For this review, take the finished solid that the model builds, in its own axes (mm). A direction names the side the tool comes from. Round coordinates to 2 decimals unless told otherwise and drop trailing zeros. Write each loop counter-clockwise with the first axis right and the second up, starting at its lowest first coordinate (ties: lowest second). Pieces come first, ordered by that corner, then holes. Notation, with made-up numbers: M 60.5,85.5 L 75.5,85.5 A20 cw 75.5,115.5 Z; hole C -4,87 d5. An arc over 180 degrees is marked long. Answer in a Markdown table with one row per item.
```python
from build123d import *

# Parameters (mm, degrees)
SKETCH1_R           = 20.32
BOSS_EXTRUDE1_DEPTH = 26.416
BOSS_EXTRUDE2_DEPTH = 6.35
SKETCH3_R           = 12.7
BOSS_EXTRUDE3_DEPTH = 19.05
SKETCH4_R           = 2.032
CUT_EXTRUDE1_DEPTH  = 10.16


with BuildPart() as part:
    # Sketch1 → Boss-Extrude1 (new body)
    with BuildSketch(Plane(origin=(0, 0, 0), x_dir=(1, 0, 0), z_dir=(0, 1, 0))):
        Circle(SKETCH1_R)
    extrude(amount=BOSS_EXTRUDE1_DEPTH)

    # Sketch2 → Boss-Extrude2 (add)
    with BuildSketch(Plane.XZ):
        Polygon((-11.878404438, 20.574), (11.878404438, 20.574), (23.756808877, 0), (11.878404438, -20.574), (-11.878404438, -20.574), (-23.756808877, 0), align=None)
    extrude(amount=BOSS_EXTRUDE2_DEPTH)

    # Sketch3 → Boss-Extrude3 (add)
    with BuildSketch(Plane(origin=(0, -6.35, 0), x_dir=(-1, 0, 0), z_dir=(0, -1, 0))):
        Circle(SKETCH3_R)
    extrude(amount=BOSS_EXTRUDE3_DEPTH)

    # Sketch4 → Cut-Extrude1 (cut)
    with BuildSketch(Plane(origin=(0, 26.416, 0), x_dir=(1, 0, 0), z_dir=(0, 1, 0))):
        with Locations((0, -12.7)):
            Circle(SKETCH4_R)
        with Locations((-12.7, 0)):
            Circle(SKETCH4_R)
        with Locations((12.7, 0)):
            Circle(SKETCH4_R)
    extrude(amount=-CUT_EXTRUDE1_DEPTH, mode=Mode.SUBTRACT)


solid = part.part
```
Q1. Mouldability with a two-part tool opening along Z and no side actions: class faces 4 (the face through (0, 16.256, 13)), 5 (the face through (-14.73, 21.41, -0.09)), 6 (the face through (0, 26.416, 0)), 7 (the face through (0, -3, 20.574)) as +Z half, -Z half, draft (parallel to the pull), parting line (faces both ways), or undercut.
Found:
| item | result |
|---|---|
| face 4 | undercut |
| face 5 | undercut |
| face 6 | draft |
| face 7 | +Z half |
Q2. Take a section at C-C (z = 8.5). State the section outline as (x, y) points, then the cut area to 3 significant figures.
Found:
| item | result |
|---|---|
| outline | M -18.85,-6.35 L -9.44,-6.35 L -9.44,-25.4 L 9.44,-25.4 L 9.44,-6.35 L 18.85,-6.35 L 18.85,0 L 18.46,0 L 18.46,26.42 L -18.46,26.42 L -18.46,0 L -18.85,0 Z |
| area | 1,570 mm² |
Q3. Machinability: for faces 1 (the face through (0, -25.4, 0)), 2 (the face through (2.75, -15.74, 12.4)), 3 (the face through (-13, 16.256, 0)), which of the approach directions +Z, -Z, +X, -X, +Y, -Y give a long, thin tool a straight path to every point of the face, cutting with its end or side? Answer none if there is none.
Found:
| item | result |
|---|---|
| face 1 | +Z, -Z, +X, -X, -Y |
| face 2 | -Y |
| face 3 | +Y |
Q4. Take a section at B-B (y = 20.5). State the section outline as (x, z) points.
Found:
| item | result |
|---|---|
| outline | C 0,0 d40.64; hole C -12.7,0 d4.06; hole C 0,12.7 d4.06; hole C 12.7,0 d4.06 |
Q5. Take a section at A-A (x = 0). State the section outline as (y, z) points, then the cut area to 3 significant figures.
Found:
| item | result |
|---|---|
| outline | M -25.4,-12.7 L -6.35,-12.7 L -6.35,-20.57 L 0,-20.57 L 0,-20.32 L 26.42,-20.32 L 26.42,10.67 L 16.26,10.67 L 16.26,14.73 L 26.42,14.73 L 26.42,20.32 L 0,20.32 L 0,20.57 L -6.35,20.57 L -6.35,12.7 L -25.4,12.7 Z |
| area | 1,780 mm² |
Q6. Insertion check: P1, Ø3, axis at x = -8.5, y = 5.5, coming from the -Z side; P2, Ø2, axis at x = -16, z = 14.5, coming from the +Y side; P3, Ø2, axis at x = -12.5, z = -0.5, coming from the +Y side. Each pin has a flat end and moves straight along its axis. Give the tip position at first contact, or say it passes through.
Found:
| item | result |
|---|---|
| P1 | z = -19.08 |
| P2 | y = 0 |
| P3 | y = 16.26 |
Q7. Take a section at D-D (y = -5). State the section outline as (x, z) points, then the cut area to 3 significant figures.
Found:
| item | result |
|---|---|
| outline | M -23.76,0 L -11.88,-20.57 L 11.88,-20.57 L 23.76,0 L 11.88,20.57 L -11.88,20.57 Z |
| area | 1,470 mm² |
Q8. For probe 1 along X at (y, z) = (20, 0); probe 2 along Z at (x, y) = (0, 19.5); probe 3 along Y at (x, z) = (15.5, -10), list the stretches that pass through material, from the lowest coordinate up.
Found:
| item | result |
|---|---|
| probe 1 | -20.32 to -14.73, -10.67 to 10.67, 14.73 to 20.32 |
| probe 2 | -20.32 to 10.67, 14.73 to 20.32 |
| probe 3 | -6.35 to 26.42 |
